Geometry: final body of the model. Coordinates: model frame, mm. A direction names the side the tool comes from. Coordinates: 2 decimals unless noted, no trailing zeros. Order: outer loops, then holes, each group sorted by start corner. A loop starts at its lowest first (then second) coordinate and runs counter-clockwise, first axis right, second up. Notation, with made-up numbers: (62, -3) -> (91, -3) arc R21 ccw to (91, 24) -> close; hole circle Ø2 at (23, -10.75). An arc over 180 degrees is marked (long way). Use one line per item in the form item = value.
```python
from build123d import *

# Parameters (mm, degrees)
SKETCH1_W           = 65
SKETCH1_H           = 35
SKETCH1_W_2         = 40
SKETCH1_H_2         = 29
BOSS_EXTRUDE1_DEPTH = 1.5
CUT_EXTRUDE1_DEPTH  = 2.5
FILLET2_R           = 1.5


with BuildPart() as part:
    # Sketch1 → Boss-Extrude1 (new body)
    with BuildSketch(Plane(origin=(0, 0, 0), x_dir=(1, 0, 0), z_dir=(0, 1, 0))):
        Rectangle(SKETCH1_W, SKETCH1_H)
        Rectangle(SKETCH1_W_2, SKETCH1_H_2, mode=Mode.SUBTRACT)
    extrude(amount=BOSS_EXTRUDE1_DEPTH)

    # Sketch2 → Cut-Extrude1 (cut, through all)
    with BuildSketch(Plane(origin=(0, 1.5, 0), x_dir=(1, 0, 0), z_dir=(0, 1, 0))):
        with BuildLine():
            Line((-31.1, -15.5), (-31.1, 15.5))
            ThreePointArc((-31.1, 15.5), (-30, 16.6), (-28.9, 15.5))
            Line((-28.9, 15.5), (-28.9, -15.5))
            ThreePointArc((-28.9, -15.5), (-30, -16.6), (-31.1, -15.5))
        make_face()
        with BuildLine():
            Line((31.1, -15.5), (31.1, 15.5))
            ThreePointArc((31.1, 15.5), (30, 16.6), (28.9, 15.5))
            Line((28.9, 15.5), (28.9, -15.5))
            ThreePointArc((28.9, -15.5), (30, -16.6), (31.1, -15.5))
        make_face()
    extrude(amount=-CUT_EXTRUDE1_DEPTH, mode=Mode.SUBTRACT)

    # Fillet2
    fillet2_edges = [part.edges().sort_by_distance(p)[0] for p in [
        (32.5, 0.75, 17.5),
        (-32.5, 0.75, 17.5),
        (-32.5, 0.75, -17.5),
        (32.5, 0.75, -17.5),
    ]]
    fillet(fillet2_edges, radius=FILLET2_R)


solid = part.part
```
1) Material intervals for probe 1 along X at (y, z) = (0.45, 11.5); probe 2 along Z at (x, y) = (5.5, 1.35); probe 3 along X at (y, z) = (0.45, -16), sorted ascending. Write a range as from..to.
Results found:
probe_1 = -32.5..-31.1, -28.9..-20, 20..28.9, 31.1..32.5
probe_2 = -17.5..-14.5, 14.5..17.5
probe_3 = -32.5..-30.98, -29.02..29.02, 30.98..32.5
2) Contact query for a flat-ended pin moving along its axis: P1, Ø10, axis at x = -12, z = -2, coming from the +Y side. Output: stop coordinate, or through.
Results found:
P1 = through
3) Pull-direction query (X, two-part tool) for faces 1 (the flat face through (21, 1.5, 0)), 2 (the cylindrical face through (30, 0.8, 16.6)), 3 (the cylindrical face through (32.05, 0.76, -17.07)), 4 (the flat face through (0, 1, -14.5)); classes: released by +X, released by -X, zero draft, split by the parting line, or undercut.
Results found:
face_1 = zero draft
face_2 = undercut
face_3 = released by +X
face_4 = undercut
4) Section B-B, the plane z = 0. Output: boundary loops of the cut face in (x, y), and give its area (3 significant figures).
Results found:
outline = (-32.5, 0) -> (-31.1, 0) -> (-31.1, 1.5) -> (-32.5, 1.5) -> close; (-28.9, 0) -> (-20, 0) -> (-20, 1.5) -> (-28.9, 1.5) -> close; (20, 0) -> (28.9, 0) -> (28.9, 1.5) -> (20, 1.5) -> close; (31.1, 0) -> (32.5, 0) -> (32.5, 1.5) -> (31.1, 1.5) -> close
area = 30.9 mm2
5) Access query for faces 5 (the flat face through (-32.5, 1, 0)), 6 (the flat face through (-28.9, 1, 0)). Directions: +Z, -Z, +X, -X, +Y, -Y. A direction counts if a zero-diameter tool reaches every point of the face in a straight line with its end or side. Return the directions, or none.
Results found:
face_5 = +Z, -Z, -X, +Y, -Y
face_6 = +Y, -Y
6) Section A-A, the plane x = -3.5. Output: boundary loops of the cut face in (y, z).
Results found:
outline = (0, -17.5) -> (1.5, -17.5) -> (1.5, -14.5) -> (0, -14.5) -> close; (0, 14.5) -> (1.5, 14.5) -> (1.5, 17.5) -> (0, 17.5) -> close
7) Section C-C, the plane x = 30. Output: boundary loops of the cut face in (y, z), and give its area (3 significant figures).
Results found:
outline = (0, -17.5) -> (1.5, -17.5) -> (1.5, -16.6) -> (0, -16.6) -> close; (0, 16.6) -> (1.5, 16.6) -> (1.5, 17.5) -> (0, 17.5) -> close
area = 2.70 mm2
